Autodesk Inventor part; units mm, degrees
ref_plane "YZ Plane" through (0, 0, 0) normal (1, 0, 0) x (0, 1, 0)
ref_plane "XZ Plane" through (0, 0, 0) normal (0, 1, 0) x (-1, 0, 0)
ref_plane "XY Plane" through (0, 0, 0) normal (0, 0, 1) x (1, 0, 0)
sketch "Sketch2" plane through (0, 0, 0) normal (0, 0, 1) x (1, 0, 0)
  line L0 (-299.9999, -180.4934) -> (300.0001, -180.4934)
  line L1 (300.0001, -180.4934) -> (300.0001, 219.5066)
  line L2 (-299.9999, 219.5066) -> (300.0001, 219.5066)
  line L3 (-299.9999, -180.4934) -> (-299.9999, 219.5066)
  line L4 (-93.75, 46) -> (-93.75, -46)
  arc A0 (-93.75, -46) -> (-81.75, -58) centre (-81.75, -46) ccw
  line L5 (-81.75, -58) -> (81.75, -58)
  arc A1 (81.75, -58) -> (93.75, -46) centre (81.75, -46) ccw
  line L6 (93.75, -46) -> (93.75, 46)
  arc A2 (93.75, 46) -> (81.75, 58) centre (81.75, 46) ccw
  line L7 (81.75, 58) -> (-81.75, 58)
  arc A3 (-81.75, 58) -> (-93.75, 46) centre (-81.75, 46) ccw
  point P0 (0, 0)
extrude "Extrusion1" add sketch "Sketch2" along normal blind 8
sketch "Sketch3" plane through (0, 0, 8) normal (0, 0, 1) x (1, 0, 0)
  arc A0 (86.75, -63) -> (98.75, -51) centre (86.75, -51) ccw
  line L0 (-86.75, -63) -> (86.75, -63)
  arc A1 (-98.75, -51) -> (-86.75, -63) centre (-86.75, -51) ccw
  line L1 (-98.75, 51) -> (-98.75, -51)
  arc A2 (-86.75, 63) -> (-98.75, 51) centre (-86.75, 51) ccw
  line L2 (86.75, 63) -> (-86.75, 63)
  arc A3 (98.75, 51) -> (86.75, 63) centre (86.75, 51) ccw
  line L3 (98.75, -51) -> (98.75, 51)
  point P0 (0, 0)
extrude "Extrusion2" cut sketch "Sketch3" against normal blind 4
sketch "Sketch4" plane through (0, 0, 8) normal (0, 0, 1) x (1, 0, 0)
  line L0 (-269.9999, -146.4934) -> (-258.9999, -146.4934)
  line L1 (-258.9999, -146.4934) -> (-258.9999, -160.4934)
  line L2 (-258.9999, -160.4934) -> (-269.9999, -160.4934)
  line L3 (-269.9999, -160.4934) -> (-269.9999, -146.4934)
  line L4 (-228.9999, -146.4934) -> (-217.9999, -146.4934)
  line L5 (-217.9999, -146.4934) -> (-217.9999, -160.4934)
  line L6 (-217.9999, -160.4934) -> (-228.9999, -160.4934)
  line L7 (-228.9999, -160.4934) -> (-228.9999, -146.4934)
  line L8 (-299.9999, 219.5066) -> (-299.9999, -180.4934)
  line L9 (-299.9999, -180.4934) -> (300.0001, -180.4934)
  line L10 (-299.9999, -131.4934) -> (-6.35, -131.4934) construction
  line L11 (-284.9999, -131.4934) -> (-284.9999, 24.5066) construction
  line L12 (-284.9999, -104.4934) -> (-276.9999, -104.4934) construction
  line L13 (-284.9999, -53.4934) -> (-276.9999, -53.4934) construction
  line L14 (-276.9999, 23.0066) -> (-276.9999, -53.4934) construction
  line L15 (-190.9999, -131.4934) -> (-190.9999, 19.5066) construction
  line L16 (-197.9999, 19.5066) -> (-197.9999, -53.4934) construction
  circle A0 centre (-199.9999, -122.4934) radius 4
  line L17 (-276.9999, -104.4934) -> (-197.9999, -104.4934)
  line L18 (-197.9999, -104.4934) -> (-6.35, -104.4934) construction
  line L19 (-197.9999, -53.4934) -> (-197.9999, -104.4934)
  line L20 (-197.9999, -53.4934) -> (-6.35, -53.4934) construction
  line L21 (-276.9999, -53.4934) -> (-197.9999, -53.4934)
  line L22 (-276.9999, -53.4934) -> (-276.9999, -104.4934)
  line L23 (-276.9999, -104.4934) -> (-276.9999, -131.4934) construction
  point P0 (0, 0)
  dimension "d4" = 30
  dimension "d5" = 20
  dimension "d6" = 14
  dimension "d7" = 11
  dimension "d8" = 30
  dimension "d9" = 11
  dimension "d10" = 15
  dimension "d11" = 15
  dimension "d12" = 27
  dimension "d13" = 51
  dimension "d14" = 8
  dimension "d15" = 94
  dimension "d16" = 79
  dimension "d17" = 8
  dimension "d19" = 85
  dimension "d20" = 9
extrude "Extrusion3" cut sketch "Sketch4" against normal through all
sketch "Sketch5" plane through (0, 0, 8) normal (0, 0, 1) x (1, 0, 0)
  line L0 (-284.9999, -43.4934) -> (-190.9999, -43.4934)
  line L1 (-190.9999, -43.4934) -> (-190.9999, -131.4934)
  line L2 (-190.9999, -131.4934) -> (-284.9999, -131.4934)
  line L3 (-284.9999, -131.4934) -> (-284.9999, -43.4934)
  line L4 (-276.9999, -104.4934) -> (-276.9999, -53.4934)
  line L5 (-276.9999, -53.4934) -> (-197.9999, -53.4934)
  line L6 (-217.9999, -160.4934) -> (-217.9999, -146.4934)
  line L7 (-217.9999, -146.4934) -> (-228.9999, -146.4934)
  line L8 (-228.9999, -146.4934) -> (-228.9999, -160.4934)
  line L9 (-228.9999, -160.4934) -> (-217.9999, -160.4934)
  circle A0 centre (-199.9999, -122.4934) radius 4
  line L10 (-258.9999, -160.4934) -> (-258.9999, -146.4934)
  line L11 (-258.9999, -146.4934) -> (-269.9999, -146.4934)
  line L12 (-269.9999, -146.4934) -> (-269.9999, -160.4934)
  line L13 (-269.9999, -160.4934) -> (-258.9999, -160.4934)
  line L14 (-276.9999, -104.4934) -> (-197.9999, -104.4934)
  line L15 (-197.9999, -104.4934) -> (-197.9999, -53.4934)
  line L16 (98.75, -51) -> (98.75, 51)
  arc A1 (98.75, 51) -> (86.75, 63) centre (86.75, 51) ccw
  line L17 (86.75, 63) -> (-86.75, 63)
  arc A2 (-86.75, 63) -> (-98.75, 51) centre (-86.75, 51) ccw
  line L18 (-98.75, 51) -> (-98.75, -51)
  arc A3 (-98.75, -51) -> (-86.75, -63) centre (-86.75, -51) ccw
  line L19 (-86.75, -63) -> (86.75, -63)
  arc A4 (86.75, -63) -> (98.75, -51) centre (86.75, -51) ccw
  line L20 (-299.9999, -180.4934) -> (-299.9999, 219.5066)
  line L21 (-299.9999, 219.5066) -> (300.0001, 219.5066)
  line L22 (300.0001, 219.5066) -> (300.0001, -180.4934)
  line L23 (300.0001, -180.4934) -> (-299.9999, -180.4934)
  line L24 (-276.9999, -53.4934) -> (-276.9999, -104.4934)
  line L25 (-197.9999, -53.4934) -> (-276.9999, -53.4934)
  point P0 (0, 0)
  dimension "d23" = 88
  dimension "d24" = 94
  dimension "d25" = 8
  dimension "d26" = 10
sketch "Sketch6" plane through (0, 0, 0) normal (0, 0, -1) x (-1, 0, 0)
  line L0 (217.9999, -146.4934) -> (217.9999, -160.4934)
  line L1 (217.9999, -160.4934) -> (228.9999, -160.4934)
  line L2 (228.9999, -160.4934) -> (228.9999, -146.4934)
  line L3 (228.9999, -146.4934) -> (217.9999, -146.4934)
  circle A0 centre (199.9999, -122.4934) radius 4
  line L4 (258.9999, -146.4934) -> (258.9999, -160.4934)
  line L5 (258.9999, -160.4934) -> (269.9999, -160.4934)
  line L6 (269.9999, -160.4934) -> (269.9999, -146.4934)
  line L7 (269.9999, -146.4934) -> (258.9999, -146.4934)
  line L8 (276.9999, -104.4934) -> (276.9999, -53.4934)
  line L9 (276.9999, -53.4934) -> (197.9999, -53.4934)
  line L10 (197.9999, -53.4934) -> (197.9999, -104.4934)
  line L11 (197.9999, -104.4934) -> (276.9999, -104.4934)
  arc A1 (-93.75, -46) -> (-81.75, -58) centre (-81.75, -46) ccw
  line L12 (-81.75, -58) -> (81.75, -58)
  arc A2 (81.75, -58) -> (93.75, -46) centre (81.75, -46) ccw
  line L13 (93.75, -46) -> (93.75, 46)
  arc A3 (93.75, 46) -> (81.75, 58) centre (81.75, 46) ccw
  line L14 (81.75, 58) -> (-81.75, 58)
  arc A4 (-81.75, 58) -> (-93.75, 46) centre (-81.75, 46) ccw
  line L15 (-93.75, 46) -> (-93.75, -46)
  line L16 (299.9999, 219.5066) -> (299.9999, -180.4934)
  line L17 (299.9999, -180.4934) -> (-300.0001, -180.4934)
  line L18 (-300.0001, -180.4934) -> (-300.0001, 219.5066)
  line L19 (-300.0001, 219.5066) -> (299.9999, 219.5066)
  line L20 (190.9999, -43.4934) -> (284.9999, -43.4934)
  line L21 (284.9999, -43.4934) -> (284.9999, -131.4934)
  line L22 (284.9999, -131.4934) -> (190.9999, -131.4934)
  line L23 (190.9999, -131.4934) -> (190.9999, -43.4934)
  point P0 (0, 0)
  dimension "d27" = 94
  dimension "d28" = 88
  dimension "d29" = 8
  dimension "d30" = 10
extrude "Extrusion4" cut sketch "Sketch6" against normal blind 3.5 contours L20 L21 L22 L23
equation "\"d9\" = d7"
properties part number "capac cu gaura" material "Wood (Cherry)"
For this review, take the finished solid that the model builds, in its own axes (mm). A direction names the side the tool comes from. Coordinates: 2 decimals unless noted, no trailing zeros. Write each loop counter-clockwise with the first axis right and the second up, starting at its lowest first coordinate (ties: lowest second). Pieces come first, ordered by that corner, then holes. Notation, with made-up numbers: (-29, 86.5) - (-5, 86.5) arc R24 ccw to (-5, 108.5) - close; hole circle Ø5 at (49, 14.5). An arc over 180 degrees is marked (long way). Answer in a Markdown table with one row per item. Add a question column.
Q1. Draft analysis for pull direction Y (two halves, no side actions). For faces 1 (the flat face through (-4, 67, 8)), 2 (the cylindrical face through (-90.14, -54.58, 1.97)), state which applies: +Y half, -Y half, draft (parallel to the pull), parting line (faces both ways), or undercut.
Q2. We need section A-A, the plane y = -96. State the section outline as (x, z) points, and give its area (3 significant figures).
Q3. For probe 1 along X at (y, z) = (35, 5); probe 2 along X at (y, z) = (-153, 3); probe 3 along Y at (x, z) = (-245, 4.75), list the stretches that pass through material, from the lowest coordinate up.
Q4. For P1, Ø1.5, axis at x = -200, y = -96.5, coming from the -Z side; P2, Ø8, axis at x = 206, y = -136.5, coming from the -Z side, all flat-tipped, find the tip position at first contact; note any pin that passes through.
Q5. We need section B-B, the plane x = -74.5. State the section outline as (y, z) points.
Q6. Tool access review of faces 3 (the cylindrical face through (-90.33, 54.39, 1.97)), 4 (the cylindrical face through (-95.33, -59.39, 6.03)), 5 (the flat face through (-237, -106, 3.5)), 6 (the flat face through (-4, 67, 0)): name each direction out of +Z, -Z, +X, -X, +Y, -Y from which nothing blocks a thin tool from reaching the whole face with its end or side.
Answer list:
| question | item | result |
|---|---|---|
| 1 | face 1 | draft |
| 1 | face 2 | undercut |
| 2 | outline | (-300, 0) - (-285, 0) - (-285, 3.5) - (-277, 3.5) - (-277, 8) - (-300, 8) - close; (-198, 3.5) - (-191, 3.5) - (-191, 0) - (300, 0) - (300, 8) - (-198, 8) - close |
| 2 | area | 4,120 mm2 |
| 3 | probe 1 | x = -300 to -98.75, 98.75 to 300 |
| 3 | probe 2 | x = -300 to -270, -259 to -229, -218 to 300 |
| 3 | probe 3 | y = -180.49 to -104.49, -53.49 to 219.51 |
| 4 | P1 | passes through |
| 4 | P2 | stops at z = 0 |
| 5 | outline | (-180.49, 0) - (-58, 0) - (-58, 4) - (-63, 4) - (-63, 8) - (-180.49, 8) - close; (58, 0) - (219.51, 0) - (219.51, 8) - (63, 8) - (63, 4) - (58, 4) - close |
| 6 | face 3 | +Z, -Z |
| 6 | face 4 | +Z |
| 6 | face 5 | -Z |
| 6 | face 6 | -Z, +X, -X, +Y, -Y |
